Autodesk Inventor part; units mm, degrees
ref_plane "YZ Plane" through (0, 0, 0) normal (1, 0, 0) x (0, 1, 0)
ref_plane "XZ Plane" through (0, 0, 0) normal (0, 1, 0) x (-1, 0, 0)
ref_plane "XY Plane" through (0, 0, 0) normal (0, 0, 1) x (1, 0, 0)
sketch "Эскиз1" plane through (0, 0, 0) normal (0, 0, 1) x (1, 0, 0)
  line L0 (17, 0) -> (17, 0)
  line L1 (6.5, 12) -> (6.5, 19.4)
  line L2 (6.5, 19.4) -> (20.4, 19.4)
  line L3 (20.4, 19.4) -> (20.4, 0)
  line L4 (0, 0) -> (0, 10)
  line L5 (17, 0) -> (17, 0)
  line L6 (6.5, 19.4) -> (6.5, 34.4)
  line L7 (6.5, 34.4) -> (11.5, 34.4)
  line L8 (11.5, 34.4) -> (15.5192, 19.4)
  line L9 (6.5, 12) -> (6.5, 0)
  line L10 (6.5, 0) -> (20.4, 0)
  point P0 (6.5, 10)
  dimension "d2" = 10
  dimension "d18" = 13
  dimension "d20" = 5
  dimension "d21" = 75
  dimension "d22" = 15
  dimension "d30" = 40.8
  dimension "d31" = 19.4
revolve "Вращение1" add sketch "Эскиз1" angle 360 about axis through (0, 0, 0) along (0, 1, 0)
sketch "Эскиз3" plane through (0, 34.4, 0) normal (0, 1, 0) x (1, 0, 0)
  line L0 (-1, 0) -> (1, 0)
  line L1 (1, 0) -> (1, 15)
  line L2 (1, 15) -> (-1, 15)
  line L3 (-1, 15) -> (-1, 0)
  point P0 (0, 0)
  point P1 (0, 0)
  dimension "d23" = 2
  dimension "d24" = 15
extrude "Выдавливание2" cut sketch "Эскиз3" against normal up to surface (15 mm away)
pattern_circular "Круговой массив2" count 6 over 360 about axis through (0, -10, 0) along (0, 1, 0) of "Выдавливание2"
sketch "Эскиз4" plane through (0, 0, 0) normal (0, -1, 0) x (1, 0, 0)
  arc A0 (-4.3498, 16.4342) -> (-16.4073, -4.4503) centre (-0.0001, 0.0001) ccw
  arc A1 (16.4071, -4.45) -> (4.3493, 16.4343) centre (-0.0001, 0.0001) ccw
  arc A2 (2.9358, 17.8261) -> (4.3493, 16.4343) centre (4.8611, 18.3678) ccw
  arc A3 (2.9358, 17.8261) -> (-2.9363, 17.826) centre (-0.0003, 17.0002) ccw
  arc A4 (-4.3498, 16.4342) -> (-2.9363, 17.826) centre (-4.8616, 18.3676) ccw
  arc A5 (-16.9058, -6.3704) -> (-16.4073, -4.4503) centre (-18.3375, -4.9739) ccw
  arc A6 (-16.9058, -6.3704) -> (-13.9698, -11.4557) centre (-14.7225, -8.5) ccw
  arc A7 (-12.0576, -11.9839) -> (-13.9698, -11.4557) centre (-13.4762, -13.394) ccw
  arc A8 (-12.0576, -11.9839) -> (12.0576, -11.9837) centre (-0.0001, 0.0001) ccw
  arc A9 (13.9697, -11.4555) -> (12.0576, -11.9837) centre (13.4761, -13.3936) ccw
  arc A10 (13.9697, -11.4555) -> (16.9057, -6.3701) centre (14.7223, -8.4998) ccw
  arc A11 (16.4071, -4.45) -> (16.9057, -6.3701) centre (18.3373, -4.9736) ccw
extrude "Выдавливание3" cut sketch "Эскиз4" against normal blind 9.4
sketch "Эскиз5" plane through (0, 0, 0) normal (0, -1, 0) x (1, 0, 0)
  circle A0 centre (0, 0) radius 8.5
  circle A1 centre (0, 0) radius 20.4
  circle A2 centre (0, 0) radius 8.9
  dimension "d34" = 17.8
extrude "Выдавливание4" add sketch "Эскиз5" along normal blind 2 contours A1
sketch "Эскиз6" plane through (0, 0, 0) normal (0, 0, 1) x (1, 0, 0)
  arc A0 (-4.445, 6.69) -> (-3.195, 5.44) centre (-3.195, 6.69) ccw
  line L0 (-4.445, 6.69) -> (-4.445, 7.35)
  arc A1 (-3.195, 8.6) -> (-4.445, 7.35) centre (-3.195, 7.35) ccw
  line L1 (-0.2632, 8.6) -> (-3.195, 8.6)
  line L2 (3.245, 8.6) -> (-0.2432, 8.6)
  arc A2 (4.495, 7.35) -> (3.245, 8.6) centre (3.245, 7.35) ccw
  line L3 (4.495, 6.69) -> (4.495, 7.35)
  arc A3 (3.245, 5.44) -> (4.495, 6.69) centre (3.245, 6.69) ccw
  line L4 (-0.0106, 8.6) -> (-0.2632, 8.6)
  line L5 (-3.195, 5.44) -> (3.245, 5.44)
  line L6 (-0.2432, 9) -> (3.245, 9)
  arc A4 (4.895, 7.35) -> (3.245, 9) centre (3.245, 7.35) ccw
  line L7 (4.895, 7.35) -> (4.895, 6.69)
  arc A5 (3.245, 5.04) -> (4.895, 6.69) centre (3.245, 6.69) ccw
  line L8 (3.245, 5.04) -> (-3.195, 5.04)
  arc A6 (-4.845, 6.69) -> (-3.195, 5.04) centre (-3.195, 6.69) ccw
  line L9 (-4.845, 6.69) -> (-4.845, 7.35)
  arc A7 (-3.195, 9) -> (-4.845, 7.35) centre (-3.195, 7.35) ccw
  line L10 (-3.195, 9) -> (-0.2632, 9)
  line L11 (-0.2432, 9) -> (-0.2632, 9)
  point P0 (0, 0)
  dimension "d37" = 1.65
  dimension "d38" = 90
  dimension "d39" = 1.65
  dimension "d42" = 4.7582
extrude "Выдавливание5" cut sketch "Эскиз6" against normal through all contours L0 A1 L1 L4 L2 A2 L3 A3 L5 A0 | L6 A4 L7 A5 L8 A6 L9 A7 L10 L11
sketch "Эскиз7" plane through (0, -2, 0) normal (0, -1, 0) x (1, 0, 0)
  arc A0 (-10.8652, -13.0746) -> (10.8651, -13.0746) centre (0, 0.0001) ccw construction
  circle A1 centre (-0.0003, 17.0002) radius 1.05
  circle A2 centre (14.7223, -8.4998) radius 1.05
  circle A3 centre (-14.7225, -8.5) radius 1.05
  circle A4 centre (-0.0003, 17.0002) radius 0.75
  circle A5 centre (14.7223, -8.4998) radius 0.75
  circle A6 centre (-14.7225, -8.5) radius 0.75
  dimension "d57" = 1.5
  dimension "d58" = 1.5
  dimension "d59" = 1.5
extrude "Выдавливание6" cut sketch "Эскиз7" against normal blind 16 contours A4 | A5 | A6
properties part number "Цанга_держатель"
Build history of the part. All positions in model axes, mm. A direction names the side the tool comes from. Give positions to 0.01 mm unless a question says otherwise; leave off trailing zeros. Loops run counter-clockwise (first coordinate to the right, second up) from the corner with the lowest first, then second, coordinate; pieces in that order, holes last. Notation, with made-up numbers: (89.5, 68) - (126.5, 68) arc R21 cw to (126.5, 103) - close; hole circle Ø9 at (19.25, 66.25). An arc over 180 degrees is marked (long way). Use a Markdown table: item, result.
(1) Pull direction X, two halves, no side cores. Call faces 1 (the face through (9, -2, -4)), 2 (the face through (9, 19.4, 5)), 3 (the face through (9.41, 8.85, 18.1)): +X half, -X half, draft (parallel to the pull), parting line (faces both ways), or undercut.
Taken from the geometry:
| item | result |
|---|---|
| face 1 | draft |
| face 2 | undercut |
| face 3 | parting line |
(2) Band-saw the part on D-D (y = 26). Give the cut face in (x, z).
Taken from the geometry:
| item | result |
|---|---|
| outline | (-12.38, -5.99) - (-6.06, -2.35) arc R6.5 cw to (-6.06, 2.35) - (-12.38, 5.99) arc R13.75 ccw to start; (-11.38, -7.72) arc R13.75 ccw to (-1, -13.71) - (-1, -6.42) arc R6.5 cw to (-5.06, -4.08) - close; (-11.38, 7.72) - (-5.06, 4.08) arc R6.5 cw to (-1, 6.42) - (-1, 13.71) arc R13.75 ccw to start; (1, -13.71) arc R13.75 ccw to (11.38, -7.72) - (5.06, -4.08) arc R6.5 cw to (1, -6.42) - close; (1, 6.42) arc R6.5 cw to (5.06, 4.08) - (11.38, 7.72) arc R13.75 ccw to (1, 13.71) - close; (6.06, -2.35) - (12.38, -5.99) arc R13.75 ccw to (12.38, 5.99) - (6.06, 2.35) arc R6.5 cw to start |
(3) Wall check: line 1 along Y through (x, z) = (12.5, 6.5); line 2 along Y through (x, z) = (-6, 9); line 3 along X through (y, z) = (11.5, 4.5). Give the ranges that are in metal, low to high.
Taken from the geometry:
| item | result |
|---|---|
| line 1 | -2 to 0, 9.4 to 19.4 |
| line 2 | -2 to 0, 9.4 to 34.4 |
| line 3 | -19.9 to -4.69, 4.69 to 19.9 |
(4) Drop flat-ended pins along their axis: pin 1 Ø0.6 at (x, z) = (0, 11) entering from +Y; pin 2 Ø4.5 at (y, z) = (26, 10.5) entering from +X; pin 3 Ø2 at (y, z) = (14.5, -8.5) entering from -X; pin 4 Ø8 at (x, z) = (0, 0) entering from +Y. Give the stop position or say it passes through.
Taken from the geometry:
| item | result |
|---|---|
| pin 1 | y = 19.4 |
| pin 2 | x = 11.16 |
| pin 3 | x = -18.97 |
| pin 4 | through |
(5) Band-saw the part on B-B (x = 0). Give the number of separate pieces and of enclosed holes in the cut face, and give its area (3 significant figures).
Taken from the geometry:
| item | result |
|---|---|
| separate pieces | 4 |
| enclosed holes | 0 |
| area | 337 mm2 |
(6) Band-saw the part on C-C (y = 2). Give the cut face in (x, z), and give its area (3 significant figures).
Taken from the geometry:
| item | result |
|---|---|
| outline | circle Ø40.8 at (0, 0); hole (-16.91, -6.37) arc R3.05 ccw to (-13.97, -11.46) arc R2 cw to (-12.06, -11.98) arc R17 ccw to (12.06, -11.98) arc R2 cw to (13.97, -11.46) arc R3.05 ccw to (16.91, -6.37) arc R2 cw to (16.41, -4.45) arc R17 ccw to (4.35, 16.43) arc R2 cw to (2.94, 17.83) arc R3.05 ccw to (-2.94, 17.83) arc R2 cw to (-4.35, 16.43) arc R17 ccw to (-16.41, -4.45) arc R2 cw to start |
| area | 352 mm2 |
(7) Band-saw the part on A-A (z = 0). Give the cut face in (x, y).
Taken from the geometry:
| item | result |
|---|---|
| outline | (-20.4, -2) - (-8.9, -2) - (-8.9, 0) - (-17, 0) - (-17, 9.4) - (-6.5, 9.4) - (-6.5, 34.4) - (-11.5, 34.4) - (-15.52, 19.4) - (-20.4, 19.4) - close; (6.5, 9.4) - (17, 9.4) - (17, 0) - (8.9, 0) - (8.9, -2) - (20.4, -2) - (20.4, 19.4) - (15.52, 19.4) - (11.5, 34.4) - (6.5, 34.4) - close |
(8) Which spindle directions (+Z, -Z, +X, -X, +Y, -Y) get a long thin tool onto all of the face, cutting with end or side? Do faces 4 (the face through (0, 5.04, -19)), 5 (the face through (-1.409, 22.075, 6.345)), 6 (the face through (15.438, -1.014, -8.275)), 7 (the face through (-3.5, 4.6, 16.9)), 8 (the face through (-9, 27.01, -4.04)). Say none if no direction does.
Taken from the geometry:
| item | result |
|---|---|
| face 4 | -Z |
| face 5 | +Y, -Y |
| face 6 | -Y |
| face 7 | none |
| face 8 | +Y |
